Autodesk Inventor part; units mm, degrees
ref_plane "YZ Plane" through (0, 0, 0) normal (1, 0, 0) x (0, 1, 0)
ref_plane "XZ Plane" through (0, 0, 0) normal (0, 1, 0) x (-1, 0, 0)
ref_plane "XY Plane" through (0, 0, 0) normal (0, 0, 1) x (1, 0, 0)
sketch "Sketch1" plane through (0, 0, 0) normal (0, 0, 1) x (1, 0, 0)
  line L0 (-5.2979, -23.5291) -> (88.6821, -23.9107)
  line L1 (88.6821, -23.9107) -> (89.0881, 76.0893)
  line L2 (89.0881, 76.0893) -> (-4.8919, 76.4709)
  line L3 (-4.8919, 76.4709) -> (-5.2979, -23.5291)
  line L4 (-5.2979, -23.5291) -> (2.9514, -23.54) construction
  circle A0 centre (26.5572, 26.3424) radius 11 construction
  circle A1 centre (41.9941, 10.7796) radius 1.5 construction
  circle A2 centre (10.9944, 10.9055) radius 1.5 construction
  circle A3 centre (11.1202, 41.9052) radius 1.5 construction
  circle A4 centre (42.12, 41.7793) radius 1.5 construction
  circle A5 centre (0.2148, 52.8996) radius 1.4224 construction
  circle A6 centre (0, 0) radius 1.4224 construction
  circle A7 centre (52.8996, -0.2148) radius 1.4224 construction
  circle A8 centre (53.1143, 52.6848) radius 1.4224 construction
  line L5 (-5.3215, -5.2784) -> (58.178, -5.5363) construction
  line L6 (58.178, -5.5363) -> (58.4358, 57.9632) construction
  line L7 (58.4358, 57.9632) -> (-5.0637, 58.221) construction
  line L8 (-5.0637, 58.221) -> (-5.3215, -5.2784) construction
  line L9 (63.369, -2.4573) -> (82.4189, -2.5346) construction
  circle A9 centre (71.5076, 7.0347) radius 1.75
  circle A10 centre (71.6629, 45.2844) radius 1.75
  circle A11 centre (71.6629, 45.2844) radius 1.75 construction
  circle A12 centre (71.5076, 7.0347) radius 1.75 construction
  point P0 (88.9156, 66.1637)
  dimension "d7" = 100
  dimension "d8" = 93.98
  dimension "d38" = 3.5
extrude "Extrusion1" add sketch "Sketch1" along normal blind 6.35
sketch "Sketch2" plane through (0, 0, 6.35) normal (0, 0, 1) x (1, 0, 0)
  circle A0 centre (0.0605, -0.0094) radius 1.4214 construction
  circle A1 centre (52.924, -0.224) radius 1.4214 construction
  circle A2 centre (53.1386, 52.6394) radius 1.4214 construction
  circle A3 centre (0.2751, 52.8541) radius 1.4214 construction
  line L0 (-5.2979, -23.5291) -> (88.6821, -23.9107) construction
  line L1 (89.0881, 76.0893) -> (-4.8919, 76.4709) construction
  line L2 (-4.8919, 76.4709) -> (-5.2979, -23.5291) construction
  line L3 (89.0881, 76.0893) -> (89.043, 64.9782)
  line L4 (89.043, 64.9782) -> (82.693, 65.004)
  line L5 (82.693, 65.004) -> (82.6479, 53.8929)
  line L6 (82.6479, 53.8929) -> (88.9978, 53.8671)
  line L7 (89.043, 64.9782) -> (88.9978, 53.8671)
  line L8 (88.9979, 53.8673) -> (88.9527, 42.7562)
  line L9 (88.9527, 42.7562) -> (82.6028, 42.782)
  line L10 (82.6028, 42.782) -> (82.5577, 31.6709)
  line L11 (82.5577, 31.6709) -> (88.9076, 31.6451)
  line L12 (88.9527, 42.7562) -> (88.9076, 31.6451)
  line L13 (88.9076, 31.6453) -> (88.8625, 20.5341)
  line L14 (88.8625, 20.5341) -> (82.5126, 20.5599)
  line L15 (82.5126, 20.5599) -> (82.4675, 9.4488)
  line L16 (82.4675, 9.4488) -> (88.8174, 9.423)
  line L17 (88.8625, 20.5341) -> (88.8174, 9.423)
  line L18 (88.8174, 9.4232) -> (88.7723, -1.6879)
  line L19 (88.7723, -1.6879) -> (82.4223, -1.6621)
  line L20 (82.4223, -1.6621) -> (82.3772, -12.7732)
  line L21 (82.3772, -12.7732) -> (88.7272, -12.799)
  line L22 (88.7723, -1.6879) -> (88.7272, -12.799)
  point P0 (0, 0)
  dimension "d12" = 6.35
  dimension "d14" = 11.1111
  dimension "d31" = 22.2222
extrude "Extrusion2" cut sketch "Sketch2" against normal blind 25.4
sketch "Sketch3" plane through (0, 0, 6.35) normal (0, 0, 1) x (1, 0, 0)
  line L0 (89.0881, 76.0893) -> (-4.8919, 76.4709) construction
  line L1 (-4.8919, 76.4709) -> (-5.2979, -23.5291) construction
  line L2 (-5.2979, -23.5291) -> (88.6821, -23.9107) construction
  line L3 (89.0881, 76.0893) -> (-4.8919, 76.4709)
  line L4 (40.0695, 76.2884) -> (40.0695, -23.7133)
  line L5 (-5.2979, -23.5291) -> (88.6821, -23.9107)
  line L6 (-4.8919, 76.4709) -> (-5.2979, -23.5291)
  point P0 (0, 0)
extrude "Extrusion3" cut sketch "Sketch3" against normal blind 25.4
equation "\"d14\" = d11"
Work out the finished part from the listing and answer in its coordinate system (mm). Give positions to 0.01 mm unless a question says otherwise; leave off trailing zeros. Loops run counter-clockwise (first coordinate to the right, second up) from the corner with the lowest first, then second, coordinate; pieces in that order, holes last. Notation, with made-up numbers: (-13, -1) -> (14, -1) arc R37 cw to (14, 36) -> close; hole circle Ø2 at (38.5, 65). An arc over 180 degrees is marked (long way). Write item = value, one per line. Start each with the question number.
(1) Find section B-B on y = 41.5. Give the vertices of the cut face in (x, z).
(2) Given pin 1 Ø3 at (x, y) = (71.51, 7.03) entering from +Z; pin 2 Ø1.5 at (x, z) = (68, 3.5) entering from +Y, each flat-ended and moving along its own axis, determine where each tip first touches the part or whether it passes through.
(3) The mould has two halves that part along Y. Classify faces 1 (the cylindrical face through (73.28, 45.95, 3.13)), 2 (the flat face through (64, 27, 0)): +Y half, -Y half, draft (parallel to the pull), parting line (faces both ways), or undercut.
(4) Find the intervals of material crossed by probe 1 along Y at (x, z) = (84.5, 2.75); probe 2 along Y at (x, z) = (70.5, 1); probe 3 along X at (y, z) = (7, 5.25), in increasing order. Write a range as from..to.
(5) Find section A-A on z = 1.75. Give the vertices of the cut face in (x, y).
From the geometry:
q1.outline = (40.07, 0) -> (82.6, 0) -> (82.6, 6.35) -> (40.07, 6.35) -> close
q2.pin_1 = through
q2.pin_2 = 76.18
q3.face_1 = undercut
q3.face_2 = draft
q4.probe_1 = -23.89..-12.78, -1.67..9.44, 20.55..31.66, 42.77..53.89, 65..76.11
q4.probe_2 = -23.84..5.6, 8.47..43.98, 46.59..76.16
q4.probe_3 = 40.07..69.76, 73.26..88.81
q5.outline = (40.07, -23.71) -> (88.68, -23.91) -> (88.73, -12.8) -> (82.38, -12.77) -> (82.42, -1.66) -> (88.77, -1.69) -> (88.82, 9.42) -> (82.47, 9.45) -> (82.51, 20.56) -> (88.86, 20.53) -> (88.91, 31.65) -> (82.56, 31.67) -> (82.6, 42.78) -> (88.95, 42.76) -> (89, 53.87) -> (82.65, 53.89) -> (82.69, 65) -> (89.04, 64.98) -> (89.09, 76.09) -> (40.07, 76.29) -> close; hole circle Ø3.5 at (71.51, 7.03); hole circle Ø3.5 at (71.66, 45.28)
